Can you work these out from the model? Positions are in its coordinate system, mm. A direction names the side the tool comes from. Give positions to 0.01 mm unless a question says otherwise; leave off trailing zeros. Order: outer loops, then holes, each group sorted by start corner. A loop starts at its lowest first (then second) coordinate and runs counter-clockwise, first axis right, second up. Notation, with made-up numbers: M 67.25,10.5 L 87.25,10.5 A29 ccw 87.25,49.5 Z; hole C -20.75,68.25 d4. An arc over 180 degrees is marked long. Write each question's results on one line, items separated by ' | '.
from build123d import *

# Parameters (mm, degrees)
F3_R     = 4.445
F4_DEPTH = 31.751


with BuildPart() as f1:
    # F0 (on Front) → F1 (revolve)
    with BuildSketch(Plane.XZ):
        Polygon((0, 26.6254378243), (0, 19.05), (38.1, 19.05), (38.1, 39.2880663276), (19.05, 39.2880663276), (19.05, 81.9719955325), (6.35, 81.9719955325), (6.35, 26.6254378243), align=None)
    revolve(axis=Axis((2.4508777199, 0, 0), (1, 0, 0)))

    # F3 (on offset) → F4 (cut, through all)
    with BuildSketch(Plane(origin=(6.35, 0, 0), x_dir=(0, -1, 0), z_dir=(-1, 0, 0))):
        with Locations((0, 54.2987166784)):
            Circle(F3_R)
        with Locations((-47.0240680364, 27.1493583392)):
            Circle(F3_R)
        with Locations((-47.0240680364, -27.1493583392)):
            Circle(F3_R)
        with Locations((0, -54.2987166784)):
            Circle(F3_R)
        with Locations((47.0240680364, -27.1493583392)):
            Circle(F3_R)
        with Locations((47.0240680364, 27.1493583392)):
            Circle(F3_R)
    extrude(amount=-F4_DEPTH, mode=Mode.SUBTRACT)


solid = f1.part
(1) Imagine slicing it at C-C, the plane x = 27. Write out the boundary of the cut face in (y, z), plus the area to 3 significant figures.
Data:
outline: C 0,0 d78.58; hole C 0,0 d38.1 | area: 3,710 mm2
(2) Imagine slicing it at B-B, the plane z = 0. Write out the boundary of the cut face in (x, y), plus the area to 3 significant figures.
Data:
outline: M 0,-26.63 L 6.35,-26.63 L 6.35,-81.97 L 19.05,-81.97 L 19.05,-39.29 L 38.1,-39.29 L 38.1,-19.05 L 0,-19.05 Z; M 0,19.05 L 38.1,19.05 L 38.1,39.29 L 19.05,39.29 L 19.05,81.97 L 6.35,81.97 L 6.35,26.63 L 0,26.63 Z | area: 2,470 mm2
(3) We'd pull the mould along Y, two halves only. Please class faces 4 (the face through (0, 11, 17)), 5 (the face through (28.442, -38.954, -5.115)), 6 (the face through (12.611, 0.579, 58.706)): +Y half, -Y half, draft (parallel to the pull), parting line (faces both ways), or undercut.
Data:
face 4: draft | face 5: parting line | face 6: undercut
(4) Imagine slicing it at A-A, the plane y = 0. Write out the boundary of the cut face in (x, z), plus the area to 3 significant figures.
Data:
outline: M 0,-26.63 L 6.35,-26.63 L 6.35,-49.85 L 19.05,-49.85 L 19.05,-39.29 L 38.1,-39.29 L 38.1,-19.05 L 0,-19.05 Z; M 0,19.05 L 38.1,19.05 L 38.1,39.29 L 19.05,39.29 L 19.05,49.85 L 6.35,49.85 L 6.35,26.63 L 0,26.63 Z; M 6.35,-81.97 L 19.05,-81.97 L 19.05,-58.74 L 6.35,-58.74 Z; M 6.35,58.74 L 19.05,58.74 L 19.05,81.97 L 6.35,81.97 Z | area: 2,240 mm2
(5) Will these pins go through, and if not, where does the flat tip stop? P1, Ø14, axis at y = 47.02, z = 27.15, coming from the +X side; P2, Ø5, axis at y = -41, z = -54, coming from the -X side; P3, Ø5, axis at x = 32.5, y = 14, coming from the -Z side.
Data:
P1: stops at x = 19.05 | P2: stops at x = 6.35 | P3: stops at z = -37.57
(6) For faces 1 (the face through (3.131, -7.998, 25.396)), 2 (the face through (12.611, 44.973, 23.206)), 3 (the face through (19.05, -19, -35)), which set-ups out of +Z, -Z, +X, -X, +Y, -Y let a thin tool reach every point of the face, with its end or its side?
Data:
face 1: -X | face 2: +X, -X | face 3: +X
(7) Imagine slicing it at D-D, the plane x = 9. Write out the boundary of the cut face in (y, z) (3 decimals), plus the area to 3 significant figures.
Data:
outline: C 0,0 d163.944; hole C -47.024,-27.149 d8.89; hole C -47.024,27.149 d8.89; hole C 0,0 d38.1; hole C 0,-54.299 d8.89; hole C 0,54.299 d8.89; hole C 47.024,-27.149 d8.89; hole C 47.024,27.149 d8.89 | area: 19,600 mm2
(8) I need wall thicknesses on L1, parallel to Z at x = 13, y = 0; L2, parallel to Z at x = 11.5, y = 3.5; L3, parallel to Z at x = 12, y = 46. Which ranges of each line are inside material? Lowest first, please. Write a range as from..to.
Data:
L1: z = -81.97..-58.74, -49.85..-19.05, 19.05..49.85, 58.74..81.97 | L2: z = -81.9..-57.04, -51.56..-18.73, 18.73..51.56, 57.04..81.9 | L3: z = -67.85..-31.47, -22.82..22.82, 31.47..67.85
